```python
from build123d import *

# Parameters (mm, degrees)
SKETCH1_W           = 14
SKETCH1_H           = 38.75
BOSS_EXTRUDE1_DEPTH = 27
SKETCH2_R           = 8.625
CUT_EXTRUDE1_DEPTH  = 15
CHAMFER1_SIZE       = 2
CHAMFER2_SIZE       = 2


with BuildPart() as part:
    # Sketch1 → Boss-Extrude1 (new body)
    with BuildSketch(Plane.XY):
        Rectangle(SKETCH1_W, SKETCH1_H)
        with BuildLine():
            ThreePointArc((2.75, -11.375), (0, -14.125), (-2.75, -11.375))
            Line((-2.75, -11.375), (-2.75, -8.625))
            Line((-2.75, -8.625), (0, -8.625))
            Line((0, -8.625), (2.75, -8.625))
            Line((2.75, -8.625), (2.75, -11.375))
        make_face(mode=Mode.SUBTRACT)
        with BuildLine():
            Line((-2.75, 8.625), (-2.75, 11.375))
            ThreePointArc((-2.75, 11.375), (0, 14.125), (2.75, 11.375))
            Line((2.75, 11.375), (2.75, 8.625))
            Line((2.75, 8.625), (0, 8.625))
            Line((0, 8.625), (-2.75, 8.625))
        make_face(mode=Mode.SUBTRACT)
    extrude(amount=BOSS_EXTRUDE1_DEPTH)

    # Sketch2 → Cut-Extrude1 (cut, through all)
    with BuildSketch(Plane.ZY.offset(7)):
        with BuildLine():
            ThreePointArc((10.625, -8.625), (2, 0), (10.625, 8.625))
            Line((10.625, 8.625), (0, 8.625))
            Line((0, 8.625), (0, 0))
            Line((0, 0), (0, -8.625))
            Line((0, -8.625), (10.625, -8.625))
        make_face()
        with Locations((10.625, 0)):
            Circle(SKETCH2_R)
    extrude(amount=-CUT_EXTRUDE1_DEPTH, mode=Mode.SUBTRACT)

    # Chamfer1
    chamfer1_edges = [part.edges().sort_by_distance(p)[0] for p in [
        (7, -19.375, 13.5),
        (-7, -19.375, 13.5),
        (-7, 19.375, 13.5),
        (7, 19.375, 13.5),
    ]]
    chamfer(chamfer1_edges, length=CHAMFER1_SIZE)

    # Chamfer2
    chamfer2_edges = [part.edges().sort_by_distance(p)[0] for p in [
        (0, -19.375, 27),
        (0, 19.375, 27),
    ]]
    chamfer(chamfer2_edges, length=CHAMFER2_SIZE)


solid = part.part
```
CAD build for the part. Positions are in the model's coordinates, mm. A direction names the side the tool comes from. Round coordinates to 2 decimals unless told otherwise and drop trailing zeros. Order: outer loops, then holes, each group sorted by start corner. A loop starts at its lowest first (then second) coordinate and runs counter-clockwise, first axis right, second up.
Q1. Slice it at C-C (z = 2.5). Write the cut outline in (x, y) (3 decimals).
Q2. Slice it at D-D (z = 16.5). Write the cut outline in (x, y) (3 decimals).
Q3. Two-plate mould, pull along Y, no slides. Class faces 4 (the flat face through (6.014, 18.361, 13.311)), 5 (the flat face through (5, -8.625, 5)), 6 (the flat face through (-2.75, 10, 13)), 7 (the flat face through (0, -19.375, 12)): pulls with the +Y half, pulls with the -Y half, needs draft (parallel to the pull), parting line crosses it, or undercut.
Q4. Slice it at A-A (x = 0). Write the cut outline in (y, z) (3 decimals).
Q5. Which spindle directions (+Z, -Z, +X, -X, +Y, -Y) get a long thin tool onto all of the face, cutting with end or side? Do faces 1 (the cylindrical face through (0.06, -14.124, 13.311)), 2 (the flat face through (-5, 8.625, 5)), 3 (the flat face through (-5.986, -18.389, 13.311)). Say none if no direction does.
Q6. Slice it at B-B (y = -10). Write the cut outline in (x, z).
Q7. Wall check: L1, parallel to Y at x = 2.5, z = 25.25 (3 decimals); L2, parallel to Y at x = 0.25, z = 15.5 (3 decimals); L3, parallel to Y at x = 1, z = 22 (3 decimals). Give the ranges that are in metal, low to high.
Results below:
1. outline: (-7, -17.375) - (-5, -19.375) - (5, -19.375) - (7, -17.375) - (7, -8.625) - (2.75, -8.625) - (2.75, -11.375) arc R2.75 cw to (-2.75, -11.375) - (-2.75, -8.625) - (-7, -8.625) - close; (-7, 8.625) - (-2.75, 8.625) - (-2.75, 11.375) arc R2.75 cw to (2.75, 11.375) - (2.75, 8.625) - (7, 8.625) - (7, 17.375) - (5, 19.375) - (-5, 19.375) - (-7, 17.375) - close
2. outline: (-7, -17.375) - (-5, -19.375) - (5, -19.375) - (7, -17.375) - (7, -6.315) - (-7, -6.315) - close; (-7, 6.315) - (7, 6.315) - (7, 17.375) - (5, 19.375) - (-5, 19.375) - (-7, 17.375) - close; hole (-2.75, -11.375) arc R2.75 ccw to (2.75, -11.375) - (2.75, -8.625) - (-2.75, -8.625) - close; hole (-2.75, 8.625) - (2.75, 8.625) - (2.75, 11.375) arc R2.75 ccw to (-2.75, 11.375) - close
3. face 4: pulls with the +Y half
3. face 5: undercut
3. face 6: undercut
3. face 7: pulls with the -Y half
4. outline: (-19.375, 0) - (-14.125, 0) - (-14.125, 27) - (-17.375, 27) - (-19.375, 25) - close; (-8.625, 10.625) arc R8.625 cw to (8.625, 10.625) - (8.625, 27) - (-8.625, 27) - close; (14.125, 0) - (19.375, 0) - (19.375, 25) - (17.375, 27) - (14.125, 27) - close
5. face 1: +Z, -Z
5. face 2: -Z, +X, -X
5. face 3: +Z, -Z, -X, -Y
6. outline: (-7, 0) - (-2.75, 0) - (-2.75, 27) - (-7, 27) - close; (2.75, 0) - (7, 0) - (7, 27) - (2.75, 27) - close
7. L1: y = -19.125 to -12.521, -8.625 to 8.625, 12.521 to 19.125
7. L2: y = -19.375 to -14.114, -8.625 to -7.115, 7.115 to 8.625, 14.114 to 19.375
7. L3: y = -19.375 to -13.937, -8.625 to 8.625, 13.937 to 19.375
